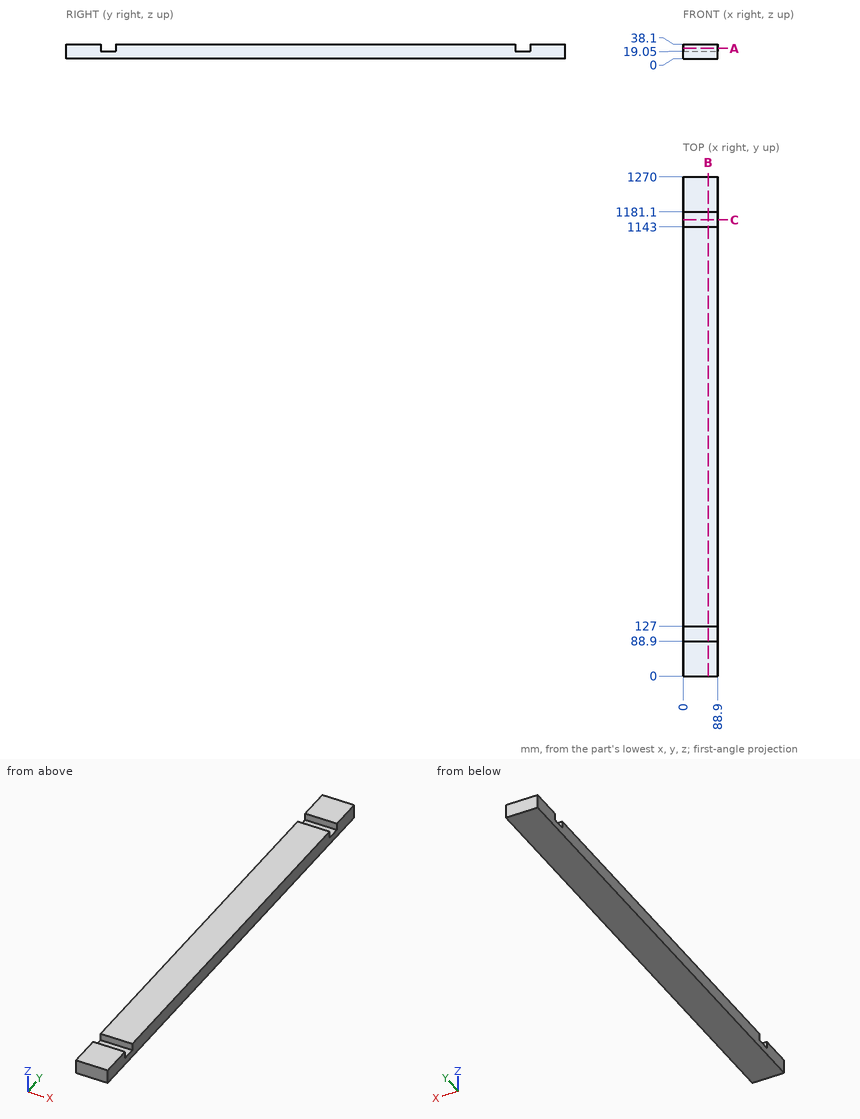
Could you check a few things on this drawing? It's one solid part, dimensions in mm from its lowest x, y, z. Give positions to 0.01 mm unless a question says otherwise; leave off trailing zeros. Order: outer loops, then holes, each group sorted by start corner. A loop starts at its lowest first (then second) coordinate and runs counter-clockwise, first axis right, second up. Notation, with made-up numbers: (-6, 58.25) -> (53, 58.25) arc R34 cw to (53, 97.25) -> close; hole circle Ø8 at (76, 70.5). An arc over 180 degrees is marked (long way). Use CSV: the item, a comma, the result in double quotes. Start each with the question number.
Item 1: Suppose I cut it at C-C (y = 1160.5). List the corners of the cut face in (x, z) for me, and give its area (3 significant figures).
Item 2: Suppose I cut it at A-A (z = 27). List the corners of the cut face in (x, y) for me, and give its area (3 significant figures).
Item 3: Suppose I cut it at B-B (x = 64). List the corners of the cut face in (y, z) for me, and give its area (3 significant figures).
Item 4: If I drill on probe 1 along Y at (x, z) = (9, 36); probe 2 along Z at (x, y) = (7.5, 1172.5), over which ranges is the centre line in solid material (lowest first)? Write a range as [from, to].
Item 5: I'm going to push flat-ended pins straight in: P1, Ø19, axis at x = 52.5, y = 113.5, coming from the +Z side; P2, Ø8, axis at y = 197, z = 33, coming from the -X side. Where does each tip first touch, or does it pass through?
Answer block:
1,outline,"(0, 0) -> (88.9, 0) -> (88.9, 19.05) -> (0, 19.05) -> close"
1,area,"1,690 mm^2"
2,outline,"(0, 0) -> (88.9, 0) -> (88.9, 88.9) -> (0, 88.9) -> close; (0, 127) -> (88.9, 127) -> (88.9, 1143) -> (0, 1143) -> close; (0, 1181.1) -> (88.9, 1181.1) -> (88.9, 1270) -> (0, 1270) -> close"
2,area,"106,000 mm^2"
3,outline,"(0, 0) -> (1270, 0) -> (1270, 38.1) -> (1181.1, 38.1) -> (1181.1, 19.05) -> (1143, 19.05) -> (1143, 38.1) -> (127, 38.1) -> (127, 19.05) -> (88.9, 19.05) -> (88.9, 38.1) -> (0, 38.1) -> close"
3,area,"46,900 mm^2"
4,probe 1,"y = [0, 88.9], [127, 1143], [1181.1, 1270]"
4,probe 2,"z = [0, 19.05]"
5,P1,"stops at z = 19.05"
5,P2,"stops at x = 0"
